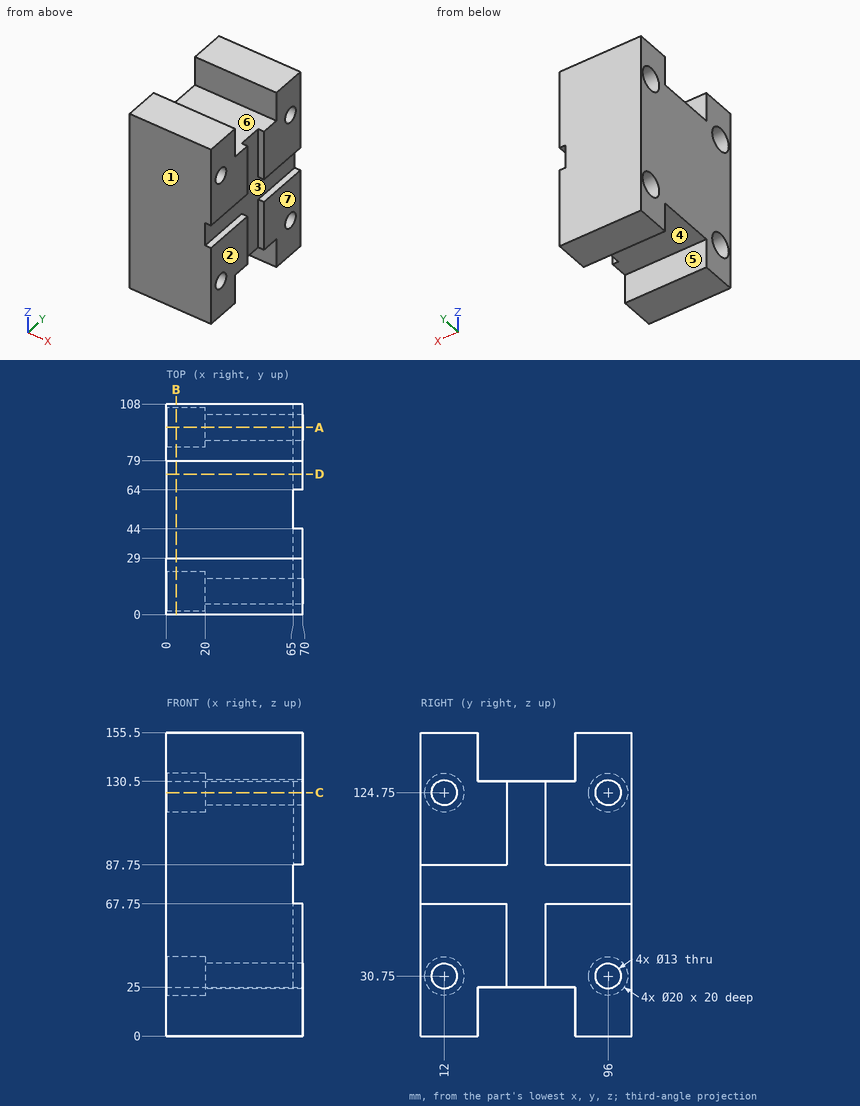
Here's the drawing with two shaded views (mm, measured from the low corner). I have some questions. A direction names the side the tool comes from. Give positions to 0.01 mm unless a question says otherwise; leave off trailing zeros. Loops run counter-clockwise (first coordinate to the right, second up) from the corner with the lowest first, then second, coordinate; pieces in that order, holes last. Notation, with made-up numbers: M 64.5,76 L 90.5,76 A38 ccw 90.5,114 Z; hole C -11,-15.75 d3. An arc over 180 degrees is marked long. Answer in a Markdown table with one row per item.
1. If I drill on line 1 along Z through (x, y) = (12, 96.5); line 2 along Z through (x, y) = (49, 12); line 3 along Y through (x, z) = (55, 142), over which ranges is the centre line in solid material (lowest first)?
Taken from the geometry:
| item | result |
|---|---|
| line 1 | z = 0 to 20.76, 40.74 to 114.76, 134.74 to 155.5 |
| line 2 | z = 0 to 24.25, 37.25 to 118.25, 131.25 to 155.5 |
| line 3 | y = 0 to 29, 79 to 108 |
2. Suppose I cut it at B-B on x = 5. Write out the boundary of the cut face in (y, z), plus the area to 3 significant figures.
Taken from the geometry:
| item | result |
|---|---|
| outline | M 0,0 L 29,0 L 29,25 L 79,25 L 79,0 L 108,0 L 108,155.5 L 79,155.5 L 79,130.5 L 29,130.5 L 29,155.5 L 0,155.5 Z; hole C 12,30.75 d20; hole C 12,124.75 d20; hole C 96,30.75 d20; hole C 96,124.75 d20 |
| area | 13,000 mm² |
3. Suppose I cut it at A-A on y = 96. Write out the boundary of the cut face in (x, z).
Taken from the geometry:
| item | result |
|---|---|
| outline | M 0,0 L 70,0 L 70,24.25 L 20,24.25 L 20,20.75 L 0,20.75 Z; M 0,40.75 L 20,40.75 L 20,37.25 L 70,37.25 L 70,67.75 L 65,67.75 L 65,87.75 L 70,87.75 L 70,118.25 L 20,118.25 L 20,114.75 L 0,114.75 Z; M 0,134.75 L 20,134.75 L 20,131.25 L 70,131.25 L 70,155.5 L 0,155.5 Z |
4. Suppose I cut it at C-C on z = 124.75. Write out the boundary of the cut face in (x, y), plus the area to 3 significant figures.
Taken from the geometry:
| item | result |
|---|---|
| outline | M 0,0 L 70,0 L 70,5.5 L 20,5.5 L 20,2 L 0,2 Z; M 0,22 L 20,22 L 20,18.5 L 70,18.5 L 70,44 L 65,44 L 65,64 L 70,64 L 70,89.5 L 20,89.5 L 20,86 L 0,86 Z; M 0,106 L 20,106 L 20,102.5 L 70,102.5 L 70,108 L 0,108 Z |
| area | 5,360 mm² |
5. Thinking about a two-plate mould opening in Y: for the marked faces 1, 2, 3 and 4, which applies, released by +Y, released by -Y, zero draft, split by the parting line, or undercut?
Taken from the geometry:
| item | result |
|---|---|
| face 1 | released by -Y |
| face 2 | zero draft |
| face 3 | undercut |
| face 4 | undercut |
6. Suppose I cut it at D-D on y = 72. Write out the boundary of the cut face in (x, z), plus the area to 4 significant figures.
Taken from the geometry:
| item | result |
|---|---|
| outline | M 0,25 L 70,25 L 70,67.75 L 65,67.75 L 65,87.75 L 70,87.75 L 70,130.5 L 0,130.5 Z |
| area | 7,285 mm² |
7. Which directions (+Z, -Z, +X, -X, +Y, -Y) give clear straight access to the entire face, cutting with the end or side of a thin tool? Please do the marked faces 5, 6 and 7.
Taken from the geometry:
| item | result |
|---|---|
| face 5 | -Z, +X, -X |
| face 6 | +Z, +X, -X |
| face 7 | +Z, -Z, +X, +Y, -Y |
8. For pin 1 Ø16 at (y, z) = (12, 30.75) entering from -X; pin 2 Ø1.5 at (x, y) = (35.5, 34) entering from +Z, each with a flat end and sliding along its axis, tell me the tip position at first contact or that it passes through.
Taken from the geometry:
| item | result |
|---|---|
| pin 1 | stops at x = 20 |
| pin 2 | stops at z = 130.5 |
